Read the model definition and answer for the solid it produces. Units are mm, in the model's axes. A direction names the side the tool comes from. Round coordinates to 2 decimals unless told otherwise and drop trailing zeros. Write each loop counter-clockwise with the first axis right and the second up, starting at its lowest first coordinate (ties: lowest second). Pieces come first, ordered by that corner, then holes.
from build123d import *

# Parameters (mm, degrees)
F0_W     = 65
F0_H     = 25
F0_R     = 2
F0_W_2   = 25
F0_H_2   = 15
F1_DEPTH = 2.5
F2_R     = 5
F3_R     = 5


with BuildPart() as f1:
    # F0 (on Top) → F1 (new body)
    with BuildSketch(Plane.XY):
        with Locations((0, 0.5)):
            Rectangle(F0_W, F0_H)
        with Locations((-17.5, 0)):
            Circle(F0_R, mode=Mode.SUBTRACT)
        with Locations((0, -1.5)):
            Rectangle(F0_W_2, F0_H_2, mode=Mode.SUBTRACT)
        with Locations((17.5, 0)):
            Circle(F0_R, mode=Mode.SUBTRACT)
    extrude(amount=F1_DEPTH)

    # F2
    f2_edges = [f1.edges().sort_by_distance(p)[0] for p in [
        (32.5, 13, 1.25),
    ]]
    fillet(f2_edges, radius=F2_R)

    # F3
    f3_edges = [f1.edges().sort_by_distance(p)[0] for p in [
        (32.5, -12, 1.25),
        (-32.5, -12, 1.25),
        (-32.5, 13, 1.25),
    ]]
    fillet(f3_edges, radius=F3_R)


solid = f1.part
Q1. Section C-C (z = 1.95) is taken. Determine the outline of the cut face in (x, y), then the cut area to 3 significant figures.
Verdict:
outline: (-32.5, -7) arc R5 ccw to (-27.5, -12) - (27.5, -12) arc R5 ccw to (32.5, -7) - (32.5, 8) arc R5 ccw to (27.5, 13) - (-27.5, 13) arc R5 ccw to (-32.5, 8) - close; hole circle Ø4 at (-17.5, 0); hole (-12.5, -9) - (12.5, -9) - (12.5, 6) - (-12.5, 6) - close; hole circle Ø4 at (17.5, 0)
area: 1,200 mm2
Q2. Which of the six approach directions +Z, -Z, +X, -X, +Y, -Y give full straight-line access (tool end or side, diameter ignored) to faces 1 (the flat face through (12.5, -2, 1)), 2 (the flat face through (0, -12, 1))?
Verdict:
face 1: +Z, -Z
face 2: +Z, -Z, +X, -X, -Y
Q3. Straight lines are drawn through the part: probe 1 along X at (y, z) = (-6.75, 0.8); probe 2 along X at (y, z) = (0.75, 2.35); probe 3 along Y at (x, z) = (-5, 1.45). For each, find the intervals that lie inside material, in ascending order.
Verdict:
probe 1: x = -32.5 to -12.5, 12.5 to 32.5
probe 2: x = -32.5 to -19.35, -15.65 to -12.5, 12.5 to 15.65, 19.35 to 32.5
probe 3: y = -12 to -9, 6 to 13
Q4. Section D-D (y = -6.25) is taken. Determine the outline of the cut face in (x, z).
Verdict:
outline: (-32.5, 0) - (-12.5, 0) - (-12.5, 2.5) - (-32.5, 2.5) - close; (12.5, 0) - (32.5, 0) - (32.5, 2.5) - (12.5, 2.5) - close
Q5. Section A-A (y = 0) is taken. Determine the outline of the cut face in (x, z), then the cut area to 3 significant figures.
Verdict:
outline: (-32.5, 0) - (-19.5, 0) - (-19.5, 2.5) - (-32.5, 2.5) - close; (-15.5, 0) - (-12.5, 0) - (-12.5, 2.5) - (-15.5, 2.5) - close; (12.5, 0) - (15.5, 0) - (15.5, 2.5) - (12.5, 2.5) - close; (19.5, 0) - (32.5, 0) - (32.5, 2.5) - (19.5, 2.5) - close
area: 80.0 mm2
Q6. Section B-B (x = 8.5) is taken. Determine the outline of the cut face in (y, z).
Verdict:
outline: (-12, 0) - (-9, 0) - (-9, 2.5) - (-12, 2.5) - close; (6, 0) - (13, 0) - (13, 2.5) - (6, 2.5) - close
